```python
from build123d import *

# Parameters (mm, degrees)
SKETCH1_W               = 50.8
SKETCH1_H               = 762
BOSS_EXTRUDE1_DEPTH     = 12.7
SHELL1_T                = -1.5875
SKETCH3_R               = 2.4892
CUT_EXTRUDE1_DEPTH      = 383.056867495
CUT_EXTRUDE2_DEPTH      = 383.056867495
CUT_EXTRUDE2_DEPTH_BACK = 383.056867495
SKETCH4_R               = 3.175
SKETCH4_R_2             = 2.4892


with BuildPart() as part:
    # Sketch1 → Boss-Extrude1 (new, symmetric)
    with BuildSketch(Plane.XY):
        Rectangle(SKETCH1_W, SKETCH1_H)
    extrude(amount=BOSS_EXTRUDE1_DEPTH, both=True)

    # Shell1
    shell1_openings = [part.faces().sort_by_distance(p)[0] for p in [
        (0, -381, 0),
        (0, 381, 0),
    ]]
    offset(amount=SHELL1_T, openings=shell1_openings, kind=Kind.INTERSECTION)

    # Sketch3 → Cut-Extrude1 (cut, symmetric)
    with BuildSketch(Plane(origin=(0, 0, 0), x_dir=(0, 0, -1), z_dir=(1, 0, 0))):
        with Locations((0, -374.65)):
            Circle(SKETCH3_R)
        with Locations((0, -361.95)):
            Circle(SKETCH3_R)
    cut_extrude1 = extrude(amount=CUT_EXTRUDE1_DEPTH, both=True, mode=Mode.SUBTRACT)

    # Sketch4 → Cut-Extrude2 (cut, two sides: drawn at the far end of the back side and taken through both)
    with BuildSketch(Plane(origin=(0, 0, 0), x_dir=(0, 0, -1), z_dir=(1, 0, 0)).offset(-CUT_EXTRUDE2_DEPTH_BACK)):
        with Locations((4.7625, 333.375)):
            Circle(SKETCH4_R)
        with Locations((4.7625, 346.075)):
            Circle(SKETCH4_R_2)
        with Locations((4.7625, 320.675)):
            Circle(SKETCH4_R_2)
    extrude(amount=CUT_EXTRUDE2_DEPTH + CUT_EXTRUDE2_DEPTH_BACK, mode=Mode.SUBTRACT)

    # Mirror1: Cut-Extrude1 across plane
    add(cut_extrude1.mirror(Plane.ZX), mode=Mode.SUBTRACT)


solid = part.part
```
Work out the finished part from the listing and answer in its coordinate system (mm). A direction names the side the tool comes from. Coordinates: 2 decimals unless noted, no trailing zeros. Loops run counter-clockwise (first coordinate to the right, second up) from the corner with the lowest first, then second, coordinate; pieces in that order, holes last.
1) Consider probe 1 along Y at (x, z) = (-24.65, 0); probe 2 along Z at (x, y) = (19.5, -49.5); probe 3 along Z at (x, y) = (-24.5, -361.95). Determine where each line is inside the solid, lowest interval first.
Results:
probe 1: y = -381 to -377.14, -372.16 to -364.44, -359.46 to 359.46, 364.44 to 372.16, 377.14 to 381
probe 2: z = -12.7 to -11.11, 11.11 to 12.7
probe 3: z = -12.7 to -2.49, 2.49 to 12.7
2) Section B-B (x = -15.5) is taken. Give the vertices of the cut face in (y, z), plus the area to 3 significant figures.
Results:
outline: (-381, -12.7) - (381, -12.7) - (381, -11.11) - (-381, -11.11) - close; (-381, 11.11) - (381, 11.11) - (381, 12.7) - (-381, 12.7) - close
area: 2,420 mm2
3) For a pull along Z with two mould halves and no side action, classify faces 3 (the flat face through (25.4, -5, 0)), 4 (the flat face through (23.812, -5, 0)), 5 (the flat face through (0, 5, -12.7)) as +Z half, -Z half, draft (parallel to the pull), parting line (faces both ways), or undercut.
Results:
face 3: draft
face 4: undercut
face 5: -Z half
4) Section A-A (y = 91) is taken. Give the vertices of the cut face in (x, z), plus the area to 3 significant figures.
Results:
outline: (-25.4, -12.7) - (25.4, -12.7) - (25.4, 12.7) - (-25.4, 12.7) - close; hole (-23.81, -11.11) - (23.81, -11.11) - (23.81, 11.11) - (-23.81, 11.11) - close
area: 232 mm2
5) For faces 1 (the flat face through (-25.4, -5, 0)), 2 (the flat face through (-23.812, -5, 0)), determine the directions among +Z, -Z, +X, -X, +Y, -Y from which every point of the face is accessible in a straight line to the end or side of a thin tool.
Results:
face 1: +Z, -Z, -X, +Y, -Y
face 2: +Y, -Y
